Can you work these out from the drawing? Everything is in mm from the part's minimum corner. A direction names the side the tool comes from. Give positions to 0.01 mm unless a question says otherwise; leave off trailing zeros. Order: outer loops, then holes, each group sorted by start corner. A loop starts at its lowest first (then second) coordinate and runs counter-clockwise, first axis right, second up. Notation, with made-up numbers: (38.25, 18.25) - (49.25, 18.25) arc R20 cw to (49.25, 43.25) - close; hole circle Ø9 at (-37, 89). An arc over 180 degrees is marked (long way). Write each question's results on one line, items separated by ' | '. Start each with the question number.
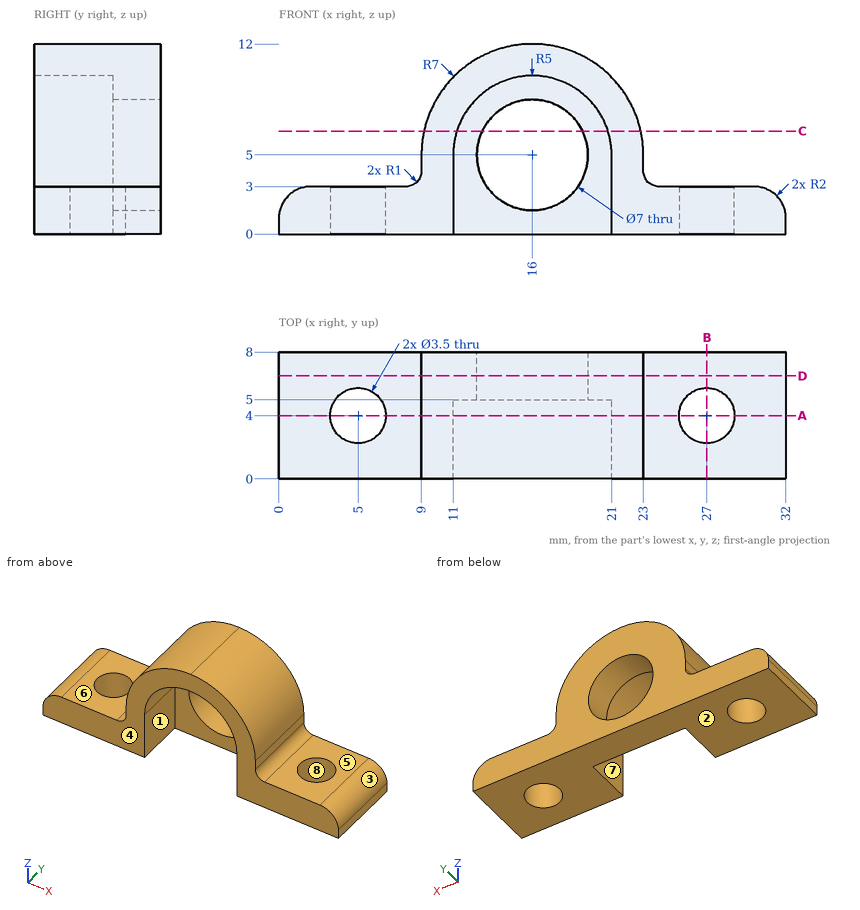
Q1. Will these pins go through, and if not, where does the flat tip stop? P1, Ø5.5, axis at x = 16, z = 5, coming from the -Y side; P2, Ø4, axis at x = 27, y = 4, coming from the +Z side; P3, Ø1.1, axis at y = 4, z = 4.5, coming from the +X side.
Q2. If we section it at A-A (y = 4): Please give me the cut outline in (x, z).
Q3. Which directions (+Z, -Z, +X, -X, +Y, -Y) give clear straight access to the entire face, cutting with the end or side of a thin tool? Please do the marked faces 4, 5, 6, 7 and 8.
Q4. If I drill on probe 1 along X at (y, z) = (4, 0.7); probe 2 along Y at (x, z) = (27, 2.2); probe 3 along X at (y, z) = (4, 1.8), over which ranges is the centre line in solid material (lowest first)? Write a range as from..to.
Q5. If we section it at D-D (y = 6.5): Please give me the cut outline in (x, z), plus the area to 3 significant figures.
Q6. Thinking about a two-plate mould opening in X: for the marked faces 1, 2 and 3, which applies, released by +X, released by -X, zero draft, split by the parting line, or undercut?
Q7. If we section it at C-C (z = 6.5): Please give me the cut outline in (x, y).
Q8. If we section it at B-B (x = 27): Please give me the cut outline in (y, z).
Findings below:
1) P1: passes through | P2: stops at z = 3 | P3: stops at x = 23
2) outline: (0, 0) - (3.25, 0) - (3.25, 3) - (2, 3) arc R2 ccw to (0, 1) - close; (6.75, 0) - (11, 0) - (11, 5) arc R5 cw to (21, 5) - (21, 0) - (25.25, 0) - (25.25, 3) - (24, 3) arc R1 cw to (23, 4) - (23, 5) arc R7 ccw to (16, 12) arc R7 ccw to (9, 5) - (9, 4) arc R1 cw to (8, 3) - (6.75, 3) - close; (28.75, 0) - (32, 0) - (32, 1) arc R2 ccw to (30, 3) - (28.75, 3) - close
3) face 4: +Z, -Z, +X, -X, -Y | face 5: +Z, +X, +Y, -Y | face 6: +Z, -X, +Y, -Y | face 7: -Z, -Y | face 8: +Z, -Z
4) probe 1: x = 0..3.25, 6.75..11, 21..25.25, 28.75..32 | probe 2: y = 0..2.25, 5.75..8 | probe 3: x = 0.17..3.25, 6.75..11, 21..25.25, 28.75..31.83
5) outline: (0, 0) - (32, 0) - (32, 1) arc R2 ccw to (30, 3) - (24, 3) arc R1 cw to (23, 4) - (23, 5) arc R7 ccw to (16, 12) arc R7 ccw to (9, 5) - (9, 4) arc R1 cw to (8, 3) - (2, 3) arc R2 ccw to (0, 1) - close; hole circle Ø7 at (16, 5) | area: 161 mm2
6) face 1: undercut | face 2: zero draft | face 3: released by +X
7) outline: (9.16, 0) - (11.23, 0) - (11.23, 5) - (12.84, 5) - (12.84, 8) - (9.16, 8) - close; (19.16, 5) - (20.77, 5) - (20.77, 0) - (22.84, 0) - (22.84, 8) - (19.16, 8) - close
8) outline: (0, 0) - (2.25, 0) - (2.25, 3) - (0, 3) - close; (5.75, 0) - (8, 0) - (8, 3) - (5.75, 3) - close
